Read the model definition and answer for the solid it produces. Units are mm, in the model's axes. Face numbers are marked on the shaded views. A direction names the side the tool comes from. Round coordinates to 2 decimals unless told otherwise and drop trailing zeros. Order: outer loops, then holes, each group sorted by start corner. A loop starts at its lowest first (then second) coordinate and runs counter-clockwise, first axis right, second up. Notation, with made-up numbers: (13.25, -20) - (47.25, -20) arc R16 ccw to (47.25, -13) - close; hole circle Ø8 at (-15.5, 43.25). An arc over 180 degrees is marked (long way). One line per question, with ' | ' between items. Start each with the question number.
1) Straight lines are drawn through the part: line 1 (X direction, y = 0, z = 10.75); line 2 (Y direction, x = 0, z = 12); line 3 (X direction, y = 14.5, z = 11.5). For each, find the intervals that lie inside material, in ascending order. Write a range as from..to.
2) The part is cut by section C-C, the plane x = 15. Give the vertices of the cut face in (y, z).
3) Flat-ended cylindrical pins translate along their axes: pin 1 (2.5 mm diameter, centred on y = 42, z = 28.5, fed in from +X); pin 2 (2 mm diameter, centred on x = -4.5, z = 20.5, fed in from +Y); pin 3 (4 mm diameter, centred on x = -4, z = 21, fed in from -Y). Find the tip coordinate at first contact, or state that the pin passes through.
4) The part is cut by section B-B, the plane y = 32. Give the vertices of the cut face in (x, z), plus the area to 3 significant figures.
5) The mould has two halves that part along X. Classify the marked faces 3, 4 and 5: pulls with the +X half, pulls with the -X half, needs draft (parallel to the pull), parting line crosses it, or undercut.
6) The part is cut by section D-D, the plane z = 19.5. Give the vertices of the cut face in (x, y), plus the area to 3 significant figures.
7) For the marked faces 1 and 2, determine the directions among +Z, -Z, +X, -X, +Y, -Y from which every point of the face is accessible in a straight line to the end or side of a thin tool.
8) The part is cut by section A-A, the plane y = 0. Give the vertices of the cut face in (x, z), plus the area to 3 significant figures.
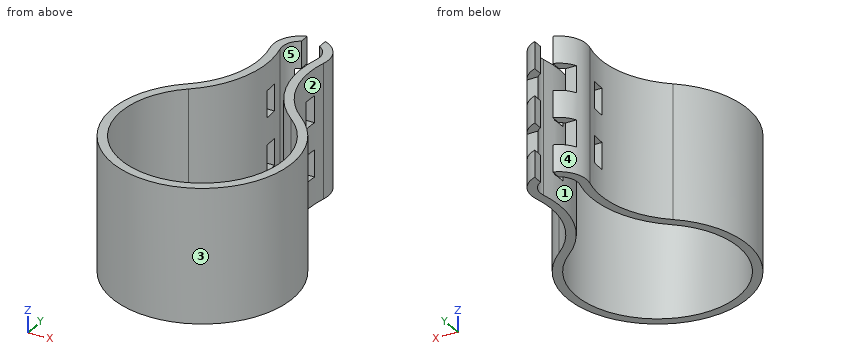
from build123d import *

# Parameters (mm, degrees)
PAD_DEPTH            = 30
SKETCH001_W          = 6
SKETCH001_H          = 3
POCKET_DEPTH         = 13.2
POCKET_DEPTH_BACK    = 13.2
SKETCH002_W          = 4
SKETCH002_H          = 4
POCKET001_DEPTH      = 30.001
SKETCH003_W          = 6
SKETCH003_H          = 3
POCKET002_DEPTH      = 13.5
POCKET002_DEPTH_BACK = 13.5


with BuildPart() as part:
    # Sketch → Pad (new body)
    with BuildSketch(Plane.XY):
        with BuildLine():
            ThreePointArc((5.9557040861, 35.8163478757), (-5.5633e-06, 43.5), (-5.9557013114, 35.8163371006))
            ThreePointArc((-12.6352136355, 15.760437062), (-6.3383082394, 24.8035240378), (-5.9557013114, 35.8163371006))
            ThreePointArc((-12.6352136355, 15.760437062), (-6.1796e-06, -20.2), (12.6352232783, 15.7604293313))
            ThreePointArc((5.9557040861, 35.8163478757), (6.3383084342, 24.8035234531), (12.6352232783, 15.7604293313))
        make_face()
        with BuildLine():
            ThreePointArc((4.018887599, 36.3150881841), (-3e-10, 41.5), (-4.0188875988, 36.3150881835))
            ThreePointArc((-11.3841995766, 14.2), (-4.4407755735, 24.1715627241), (-4.0188875988, 36.3150881835))
            ThreePointArc((-11.3841995766, 14.2), (1.86e-08, -18.2), (11.3841995475, 14.2000000233))
            ThreePointArc((4.018887599, 36.3150881841), (4.4407755675, 24.1715627421), (11.3841995475, 14.2000000233))
        make_face(mode=Mode.SUBTRACT)
    extrude(amount=PAD_DEPTH)

    # Sketch001 (on DatumPlane) → Pocket (cut, two sides)
    with BuildSketch(Plane(origin=(-1.1243e-06, 28.9018483533, 15), x_dir=(0, 0, 1), z_dir=(1, 2.57e-08, 0))) as pocket_sk:
        with Locations((-6, -2.7981516467)):
            Rectangle(SKETCH001_W, SKETCH001_H)
        with Locations((6, -2.7981516467)):
            Rectangle(SKETCH001_W, SKETCH001_H)
    extrude(amount=-POCKET_DEPTH, mode=Mode.SUBTRACT)
    extrude(pocket_sk.sketch, amount=POCKET_DEPTH_BACK, mode=Mode.SUBTRACT)

    # Sketch002 (on Face5 of Pocket) → Pocket001 (cut, through all)
    with BuildSketch(Plane.XY.offset(30)):
        with Locations((0, 42.5)):
            Rectangle(SKETCH002_W, SKETCH002_H)
    extrude(amount=-POCKET001_DEPTH, mode=Mode.SUBTRACT)

    # Sketch003 (on DatumPlane) → Pocket002 (cut, two sides)
    with BuildSketch(Plane(origin=(-1.1243e-06, 28.9018483533, 15), x_dir=(0, 0, 1), z_dir=(1, 2.57e-08, 0))) as pocket002_sk:
        with Locations((-6, -12.7638630738)):
            Rectangle(SKETCH003_W, SKETCH003_H)
        with Locations((6, -12.7638630738)):
            Rectangle(SKETCH003_W, SKETCH003_H)
    extrude(amount=-POCKET002_DEPTH, mode=Mode.SUBTRACT)
    extrude(pocket002_sk.sketch, amount=POCKET002_DEPTH_BACK, mode=Mode.SUBTRACT)


solid = part.part
Values:
1) line 1: x = -20.2..-18.2, 18.2..20.2 | line 2: y = -20.2..-18.2 | line 3: x = -14.06..-11.02, 11.02..14.06
2) outline: (-13.53, 0) - (-10.31, 0) - (-10.31, 30) - (-13.53, 30) - close; (10.31, 0) - (13.53, 0) - (13.53, 30) - (10.31, 30) - close
3) pin 1: stops at x = 5.12 | pin 2: stops at y = 40.17 | pin 3: stops at y = -20.1
4) outline: (-5.37, 0) - (-3.37, 0) - (-3.37, 6) - (-5.37, 6) - close; (-5.37, 12) - (-3.37, 12) - (-3.37, 18) - (-5.37, 18) - close; (-5.37, 24) - (-3.37, 24) - (-3.37, 30) - (-5.37, 30) - close; (3.37, 0) - (5.37, 0) - (5.37, 6) - (3.37, 6) - close; (3.37, 12) - (5.37, 12) - (5.37, 18) - (3.37, 18) - close; (3.37, 24) - (5.37, 24) - (5.37, 30) - (3.37, 30) - close | area: 72.1 mm^2
5) face 3: parting line crosses it | face 4: pulls with the -X half | face 5: undercut
6) outline: (-12.64, 15.76) arc R20.2 ccw (long way) to (12.64, 15.76) arc R19.48 cw to (5.36, 30.2) - (3.35, 30.2) arc R21.48 ccw to (11.38, 14.2) arc R18.2 cw (long way) to (-11.38, 14.2) arc R21.48 ccw to (-3.35, 30.2) - (-5.36, 30.2) arc R19.48 cw to start; (-5.96, 35.82) arc R19.48 cw to (-5.47, 33.2) - (-3.46, 33.2) arc R21.48 ccw to (-4.02, 36.32) arc R4.15 cw to (-3.05, 40.17) - (-5.47, 40.17) arc R6.15 ccw to start; (3.05, 40.17) arc R4.15 cw to (4.02, 36.32) arc R21.48 ccw to (3.46, 33.2) - (5.47, 33.2) arc R19.48 cw to (5.96, 35.82) arc R6.15 ccw to (5.47, 40.17) - close | area: 288 mm^2
7) face 1: +Z, -Z | face 2: +Z, -Z, +X
8) outline: (-20.2, 0) - (-18.2, 0) - (-18.2, 30) - (-20.2, 30) - close; (18.2, 0) - (20.2, 0) - (20.2, 30) - (18.2, 30) - close | area: 120 mm^2
